from build123d import *

# Parameters (mm, degrees)
SKETCH_1_W          = 170
SKETCH_1_H          = 85
EXTRUDE_1_DEPTH     = 65
SKETCH_2_R          = 18.25
CUT_EXTRUDE_1_DEPTH = 18
SKETCH_3_R          = 2.4
CUT_EXTRUDE_2_DEPTH = 15
FILLET_1_R          = 3


with BuildPart() as part:
    # Эскиз1 → Бобышка-Вытянуть1 (new body)
    with BuildSketch(Plane(origin=(0, 0, 0), x_dir=(1, 0, 0), z_dir=(0, 1, 0))):
        Rectangle(SKETCH_1_W, SKETCH_1_H)
    extrude(amount=EXTRUDE_1_DEPTH)

    # Эскиз2 → Вырез-Вытянуть1 (cut)
    with BuildSketch(Plane(origin=(0, 65, 0), x_dir=(1, 0, 0), z_dir=(0, 1, 0))):
        with Locations((-42.5, 0)):
            Circle(SKETCH_2_R)
        with Locations((42.5, 0)):
            Circle(SKETCH_2_R)
    extrude(amount=-CUT_EXTRUDE_1_DEPTH, mode=Mode.SUBTRACT)

    # Эскиз3 → Вырез-Вытянуть2 (cut)
    with BuildSketch(Plane(origin=(0, 47, 0), x_dir=(1, 0, 0), z_dir=(0, 1, 0))):
        with Locations((-52, 0)):
            Circle(SKETCH_3_R)
        with Locations((-33, 0)):
            Circle(SKETCH_3_R)
        with Locations((33, 0)):
            Circle(SKETCH_3_R)
        with Locations((52, 0)):
            Circle(SKETCH_3_R)
    extrude(amount=-CUT_EXTRUDE_2_DEPTH, mode=Mode.SUBTRACT)

    # Скругление1
    fillet_1_edges = [part.edges().sort_by_distance(p)[0] for p in [
        (85, 65, 0),
        (0, 65, -42.5),
        (-85, 65, 0),
        (0, 65, 42.5),
        (-85, 32.5, -42.5),
        (85, 32.5, -42.5),
        (85, 32.5, 42.5),
        (-85, 32.5, 42.5),
    ]]
    fillet(fillet_1_edges, radius=FILLET_1_R)


solid = part.part
Could you check a few things on this model? Use its own coordinates, in mm. A direction names the side the tool comes from. Coordinates: 2 decimals unless noted, no trailing zeros. Order: outer loops, then holes, each group sorted by start corner. A loop starts at its lowest first (then second) coordinate and runs counter-clockwise, first axis right, second up.
Q1. Thinking about a two-plate mould opening in X: for faces 3 (the flat face through (85, 31, 1)), 4 (the cylindrical face through (-35.398, 39.605, -0.106)), 5 (the flat face through (-1, 31, -42.5)), 6 (the flat face through (-85, 31, 1)), which applies, released by +X, released by -X, zero draft, split by the parting line, or undercut?
Q2. Will these pins go through, and if not, where does the flat tip stop? pin 1 (3 mm diameter, centred on x = 33, z = 0, fed in from -Y); pin 2 (4 mm diameter, centred on x = 33, z = 0.5, fed in from +Y); pin 3 (2.5 mm diameter, centred on x = -52, z = -1, fed in from +Y).
Q3. Which directions (+Z, -Z, +X, -X, +Y, -Y) give clear straight access to the entire face, cutting with the end or side of a thin tool? Please do faces 1 (the flat face through (-1, 31, 42.5)), 2 (the flat face through (-33, 32, 0)).
Q4. Suppose I cut it at B-B on x = -42.5. Please give me the cut outline in (y, z), and give its area (3 significant figures).
Q5. Please list where these lines run through material, in increasing order: L1, parallel to X at y = 39.25, z = 0; L2, parallel to X at y = 59.75, z = 0; L3, parallel to Z at x = -52, y = 40.
Answer:
1. face 3: released by +X
1. face 4: undercut
1. face 5: zero draft
1. face 6: released by -X
2. pin 1: stops at y = 0
2. pin 2: stops at y = 47
2. pin 3: stops at y = 32
3. face 1: +Z, +X, -X, +Y, -Y
3. face 2: +Y
4. outline: (0, -42.5) - (62, -42.5) arc R3 ccw to (65, -39.5) - (65, -18.25) - (47, -18.25) - (47, 18.25) - (65, 18.25) - (65, 39.5) arc R3 ccw to (62, 42.5) - (0, 42.5) - close
4. area: 4,860 mm2
5. L1: x = -85 to -54.4, -49.6 to -35.4, -30.6 to 30.6, 35.4 to 49.6, 54.4 to 85
5. L2: x = -85 to -60.75, -24.25 to 24.25, 60.75 to 85
5. L3: z = -42.5 to -2.4, 2.4 to 42.5
